from build123d import *

# Parameters (mm, degrees)
SKETCH010_W     = 45
SKETCH010_H     = 45
PAD002_DEPTH    = 5
SKETCH011_R     = 1
POCKET008_DEPTH = 5
SKETCH012_R     = 2
POCKET009_DEPTH = 2


with BuildPart() as part:
    # Sketch010 → Pad002 (new body)
    with BuildSketch(Plane.XY):
        with Locations((22.5, 17.5)):
            Rectangle(SKETCH010_W, SKETCH010_H)
    extrude(amount=-PAD002_DEPTH)

    # Sketch011 (on Face6 of Pad002) → Pocket008 (cut)
    with BuildSketch(Plane(origin=(0, 0, -5), x_dir=(1, 0, 0), z_dir=(0, 0, -1))):
        with Locations((10, 2.5)):
            Circle(SKETCH011_R)
        with Locations((35, 2.5)):
            Circle(SKETCH011_R)
    extrude(amount=-POCKET008_DEPTH, mode=Mode.SUBTRACT)

    # Sketch012 (on Face5 of Pocket008) → Pocket009 (cut)
    with BuildSketch(Plane(origin=(0, 0, -5), x_dir=(1, 0, 0), z_dir=(0, 0, -1))):
        with Locations((10, 2.5)):
            Circle(SKETCH012_R)
        with Locations((35, 2.5)):
            Circle(SKETCH012_R)
    extrude(amount=-POCKET009_DEPTH, mode=Mode.SUBTRACT)


solid = part.part
Input: part model. Units: mm. Frame: model coordinates. A direction names the side the tool comes from. Coordinates: 2 decimals unless noted, no trailing zeros. Loops run counter-clockwise (first coordinate to the right, second up) from the corner with the lowest first, then second, coordinate; pieces in that order, holes last.
Q1. Set-up query: faces 1 (the face through (10.9, -1.6, -3)), 2 (the face through (22, 18, -5)). Return all of +Z, -Z, +X, -X, +Y, -Y with unobstructed straight access to the full face (end or side cutting, diameter ignored); none if empty.
Q2. Contact query for flat-ended pins moving along their axis: pin 1 (1.2 mm diameter, centred on x = 10, y = -2.5, fed in from +Z); pin 2 (3 mm diameter, centred on x = 35, y = -2.5, fed in from -Z). Output: stop coordinate, or through.
Q3. Cut plane A-A (y = -2.5). Output: boundary loops of the cut face in (x, z), then the cut area to 3 significant figures.
Q4. Draft query along Y for faces 3 (the face through (0, 17, -2)), 4 (the face through (22, 40, -2)), 5 (the face through (35.954, -2.8, -1.521)). Return one class per face: +Y half, -Y half, draft (parallel to the pull), parting line (faces both ways), or undercut.
Q5. Material intervals for line 1 (X direction, y = -2.5, z = -0.75); line 2 (X direction, y = -2.5, z = -4.45); line 3 (Y direction, x = 35, z = -0.65), sorted ascending.
Q6. Cut plane B-B (x = 10). Output: boundary loops of the cut face in (y, z), then the cut area to 3 significant figures.
Working result:
1. face 1: -Z
1. face 2: -Z, +X, -X, +Y, -Y
2. pin 1: passes through
2. pin 2: stops at z = -3
3. outline: (0, -5) - (8, -5) - (8, -3) - (9, -3) - (9, 0) - (0, 0) - close; (11, -3) - (12, -3) - (12, -5) - (33, -5) - (33, -3) - (34, -3) - (34, 0) - (11, 0) - close; (36, -3) - (37, -3) - (37, -5) - (45, -5) - (45, 0) - (36, 0) - close
3. area: 197 mm2
4. face 3: draft
4. face 4: +Y half
4. face 5: undercut
5. line 1: x = 0 to 9, 11 to 34, 36 to 45
5. line 2: x = 0 to 8, 12 to 33, 37 to 45
5. line 3: y = -5 to -3.5, -1.5 to 40
6. outline: (-5, -5) - (-4.5, -5) - (-4.5, -3) - (-3.5, -3) - (-3.5, 0) - (-5, 0) - close; (-1.5, -3) - (-0.5, -3) - (-0.5, -5) - (40, -5) - (40, 0) - (-1.5, 0) - close
6. area: 211 mm2
